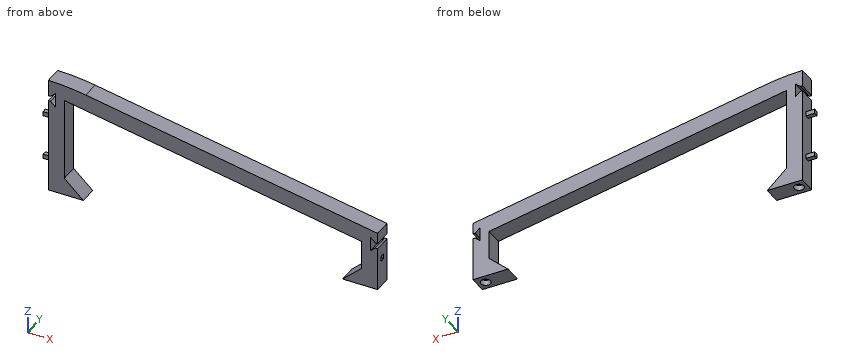
from build123d import *

# Parameters (mm, degrees)
P_IDAT_VYSUNUT_M1_DEPTH  = 8
ODEBRAT_VYSUNUT_M1_DEPTH = 161.106285011
SKICA3_W                 = 2
SKICA3_H                 = 2
P_IDAT_VYSUNUT_M2_DEPTH  = 4
SKICA5_W                 = 16
SKICA5_H                 = 8
P_IDAT_VYSUNUT_M3_DEPTH  = 8
ODEBRAT_VYSUNUT_M4_DEPTH = 161.106285011
SKICA4_W                 = 2.4
SKICA4_H                 = 2.4
ODEBRAT_VYSUNUT_M2_DEPTH = 4.4
ODEBRAT_VYSUNUT_M5_DEPTH = 161.106285011
ODEBRAT_VYSUNUT_M6_DEPTH = 161.106285011
ZAOBLIT1_R               = 100
SKICA11_R                = 2.2
ODEBRAT_VYSUNUT_M7_DEPTH = 2.4
SKICA12_R                = 1.85
ODEBRAT_VYSUNUT_M8_DEPTH = 7


with BuildPart() as part:
    # Skica1 → Přidat vysunutím1 (new body)
    with BuildSketch(Plane(origin=(0, 0, 0), x_dir=(1, 0, 0), z_dir=(0, 1, 0))):
        Polygon((0, 0), (0, -55), (150.15, -27.472114866), (150.15, 0), (142.85, 0), (142.85, -21.185463454), (7.3, -46.036644473), (7.3, 0), align=None)
    extrude(amount=P_IDAT_VYSUNUT_M1_DEPTH)

    # Skica2 → Odebrat vysunutím1 (cut, through all)
    with BuildSketch(Plane(origin=(0, 8, 0), x_dir=(1, 0, 0), z_dir=(0, 1, 0))):
        Polygon((0, -43.6), (1, -43.6), (3.2, -41.6), (3.2, -48), (1, -46), (0, -46), align=None)
    extrude(amount=-ODEBRAT_VYSUNUT_M1_DEPTH, mode=Mode.SUBTRACT)

    # Skica3 → Přidat vysunutím2 (add)
    with BuildSketch(Plane.ZY):
        with Locations((13.3, 4)):
            Rectangle(SKICA3_W, SKICA3_H)
        with Locations((34.1, 4)):
            Rectangle(SKICA3_W, SKICA3_H)
    extrude(amount=P_IDAT_VYSUNUT_M2_DEPTH)

    # Skica5 → Přidat vysunutím3 (add)
    with BuildSketch(Plane(origin=(0, 8, 0), x_dir=(1, 0, 0), z_dir=(0, 1, 0))):
        with Locations((8, -4)):
            Rectangle(SKICA5_W, SKICA5_H)
        with Locations((142.15, -4)):
            Rectangle(SKICA5_W, SKICA5_H)
    extrude(amount=-P_IDAT_VYSUNUT_M3_DEPTH)

    # Skica7 → Odebrat vysunutím4 (cut, through all)
    with BuildSketch(Plane.XZ):
        Polygon((7.3, 8), (16, 0), (16, 8), align=None)
        Polygon((134.15, 0), (134.15, 8), (142.85, 8), align=None)
    extrude(amount=-ODEBRAT_VYSUNUT_M4_DEPTH, mode=Mode.SUBTRACT)

    # Skica4 → Odebrat vysunutím2 (cut)
    with BuildSketch(Plane(origin=(150.15, 0, 0), x_dir=(0, 0, -1), z_dir=(1, 0, 0))):
        with Locations((-13.2, 4)):
            Rectangle(SKICA4_W, SKICA4_H)
    extrude(amount=-ODEBRAT_VYSUNUT_M2_DEPTH, mode=Mode.SUBTRACT)

    # Skica8 → Odebrat vysunutím5 (cut, through all)
    with BuildSketch(Plane(origin=(0, 8, 0), x_dir=(1, 0, 0), z_dir=(0, 1, 0))):
        Polygon((150.15, -20), (149.15, -20), (146.95, -18), (146.95, -24.4), (149.15, -22.4), (150.15, -22.4), align=None)
    extrude(amount=-ODEBRAT_VYSUNUT_M5_DEPTH, mode=Mode.SUBTRACT)

    # Skica9 → Odebrat vysunutím6 (cut, through all)
    with BuildSketch(Plane(origin=(0, 8, 0), x_dir=(1, 0, 0), z_dir=(0, 1, 0))):
        Polygon((0, -53.5), (8.181703712, -53.5), (0, -55), align=None)
    extrude(amount=-ODEBRAT_VYSUNUT_M6_DEPTH, mode=Mode.SUBTRACT)

    # Zaoblit1
    # the kernel refuses this fillet: 100 mm, written as the material it takes off along each edge
    with BuildSketch(Plane(origin=(8.181703712, 30.667234564, 53.5), x_dir=(0.9836061098745081, 0, -0.18033030975833525), z_dir=(0, -1, 0))) as zaoblit1_piece_1:
        with BuildLine():
            CenterArc((9.066893825, -100), ZAOBLIT1_R, 90, 9.854379591)
            Line((-8.047573761, -1.475409165), (-8.389863112, 0.495082652))
            ThreePointArc((-8.389863112, 0.495082652), (-4.3844475, 1.229507637), (-0.36066062, 1.96721222))
            Line((-0.36066062, 1.96721222), (0, 2))
            Line((0, 2), (9.066893825, 2))
            Line((9.066893825, 2), (9.066893825, 0))
        make_face()
    extrude(amount=53.334469127, mode=Mode.SUBTRACT)

    # Skica11 → Odebrat vysunutím7 (cut)
    with BuildSketch(Plane(origin=(0, 0, 0), x_dir=(-1, 0, 0), z_dir=(0, 0, -1))):
        with Locations((-146.5, 4)):
            Circle(SKICA11_R)
        with Locations((-3.65, 4)):
            Circle(SKICA11_R)
    extrude(amount=-ODEBRAT_VYSUNUT_M7_DEPTH, mode=Mode.SUBTRACT)

    # Skica12 → Odebrat vysunutím8 (cut)
    with BuildSketch(Plane(origin=(0, 0, 2.4), x_dir=(-1, 0, 0), z_dir=(0, 0, -1))):
        with Locations((-146.5, 4)):
            Circle(SKICA12_R)
        with Locations((-3.65, 4)):
            Circle(SKICA12_R)
    extrude(amount=-ODEBRAT_VYSUNUT_M8_DEPTH, mode=Mode.SUBTRACT)


solid = part.part
The listing builds one solid part. Answer for the finished solid, in the listing's coordinates (mm). Coordinates: 2 decimals unless noted, no trailing zeros. Order: outer loops, then holes, each group sorted by start corner. A loop starts at its lowest first (then second) coordinate and runs counter-clockwise, first axis right, second up. Notation, with made-up numbers: M 74.25,-18 L 87.25,-18 A20 ccw 87.25,-5 Z; hole C 76.25,47 d1. An arc over 180 degrees is marked long. Use CSV: the item, a comma, the result in double quotes.
Q1. Straight lines are drawn through the part: L1, parallel to Y at x = 3.65, z = 8; L2, parallel to Y at x = 146.5, z = 0.85; L3, parallel to X at y = 2, z = 20.5. For each, find the intervals that lie inside material, in ascending order.
Here are the results:
L1,"0 to 2.15, 5.85 to 8"
L2,"0 to 1.8, 6.2 to 8"
L3,"0 to 7.3, 142.85 to 146.95"
Q2. Section A-A (z = 5.5) is taken. Determine the outline of the cut face in (x, y), then the cut area to 3 significant figures.
Here are the results:
outline,"M 0,0 L 10.02,0 L 10.02,8 L 0,8 Z; M 140.13,0 L 150.15,0 L 150.15,8 L 140.13,8 Z; hole C 3.65,4 d3.7; hole C 146.5,4 d3.7"
area,"139 mm2"
Q3. Section C-C (z = 30) is taken. Determine the outline of the cut face in (x, y).
Here are the results:
outline,"M 0,0 L 7.3,0 L 7.3,8 L 0,8 Z; M 94.77,0 L 136.36,0 L 136.36,8 L 94.77,8 Z"
Q4. Given pin 1 Ø3 at (y, z) = (5.5, 27.5) entering from -X; pin 2 Ø3.5 at (x, y) = (146.5, 4) entering from -Z; pin 3 Ø0.6 at (x, z) = (-2.5, 13.5) entering from -Y, each flat-ended and moving along its own axis, determine where each tip first touches the part or whether it passes through.
Here are the results:
pin 1,"x = 0"
pin 2,"z = 9.4"
pin 3,"y = 3"
Q5. Section B-B (x = 139.5) is taken. Determine the outline of the cut face in (y, z).
Here are the results:
outline,"M 0,0 L 8,0 L 8,4.92 L 0,4.92 Z; M 0,21.8 L 8,21.8 L 8,29.42 L 0,29.42 Z"
Q6. Section D-D (x = 37.5) is taken. Determine the outline of the cut face in (y, z), then the cut area to 3 significant figures.
Here are the results:
outline,"M 0,40.5 L 8,40.5 L 8,48.12 L 0,48.12 Z"
area,"61.0 mm2"
